Build history of the part. All positions in model axes, mm. A direction names the side the tool comes from. Round coordinates to 2 decimals unless told otherwise and drop trailing zeros. Order: outer loops, then holes, each group sorted by start corner. A loop starts at its lowest first (then second) coordinate and runs counter-clockwise, first axis right, second up. Notation, with made-up numbers: M 9.5,8.25 L 63.5,8.25 A32 cw 63.5,44.25 Z; hole C 8,-21 d2. An arc over 180 degrees is marked long. One line per item, written item: value. Start each with the question number.
Item 1: Band-saw the part on C-C, the plane z = 10.5. Give the number of separate pieces and of enclosed holes in the cut face, then the cut area to 3 significant figures.
Item 2: Tool access for faces 4 (the flat face through (19, -16, 9.525)), 5 (the flat face through (27.99, -7.01, 35.22)), 6 (the flat face through (12.7, -8, 23)): list every direction of +Z, -Z, +X, -X, +Y, -Y with a clear straight run to the whole face (end or side of a thin tool).
Item 3: Band-saw the part on B-B, the plane z = 5.5. Write the cut outline in (x, y).
Item 4: Two-plate mould, pull along X, no slides. Class faces 1 (the flat face through (11.1, -22.23, 26.97)), 2 (the flat face through (12.7, -15, 21)), 3 (the flat face through (14, -32.4, 15.8)): +X half, -X half, draft (parallel to the pull), parting line (faces both ways), or undercut.
Item 5: Probe L1, parallel to X at y = -7.5, z = 15; L2, parallel to Y at x = 10.5, z = 24.5; L3, parallel to Y at x = 13, z = 28. List the from-to ranges inside material, lowest first.
Item 6: Band-saw the part on A-A, the plane x = 3.5. Write the cut outline in (y, z) (3 decimals).
Item 7: Band-saw the part on D-D, the plane y = -32.5. Write the cut outline in (x, z) (3 decimals).
Item 8: Pin check, flat tips, straight feed: pin 1 (3 mm diameter, centred on x = 20.5, y = -32.5, fed in from -Z) (3 decimals); pin 2 (1 mm diameter, centred on y = -31.5, z = 13, fed in from -X); pin 3 (2.5 mm diameter, centred on y = -28.5, z = 27.5, fed in from -X); pin 4 (10 mm diameter, centred on x = 28.5, y = -24, fed in from -Z). Stop position of each tip, or through.
```python
from build123d import *

# Parameters (mm, degrees)
F0_W      = 38.1
F0_H      = 37.973095
F1_DEPTH  = 38.1
F6_DEPTH  = 38.1
F8_DEPTH  = 38.1
F9_W      = 25.4
F9_H      = 7.62
F10_DEPTH = 38.1


with BuildPart() as f1:
    # F0 (on Front) → F1 (new body)
    with BuildSketch(Plane.XZ):
        with Locations((19.05, 18.986548)):
            Rectangle(F0_W, F0_H)
    extrude(amount=F1_DEPTH)

    # F5 (on offset) → F6 (cut)
    with BuildSketch(Plane.YZ.offset(38.1)):
        Polygon((-11.43, 15.875), (-6.35, 38.1), (-31.75, 38.1), (-26.67, 15.875), (-21.59, 28.575), (-16.51, 28.575), align=None)
        Polygon((-6.35, 0), (0, 0), (0, 38.1), align=None)
        Polygon((-25.4, 0), (-12.7, 0), (-19.05, 15.875), align=None)
        Polygon((-31.75, 0), (-38.1, 38.1), (-38.1, 0), align=None)
    extrude(amount=-F6_DEPTH, mode=Mode.SUBTRACT)

    # F7 (on offset) → F8 (cut)
    with BuildSketch(Plane.XZ.offset(38.1)):
        Polygon((11.43, 22.225), (6.35, 0), (31.75, 0), (26.67, 22.225), (21.59, 9.525), (16.51, 9.525), align=None)
        Polygon((25.4, 38.1), (12.7, 38.1), (19.05, 22.225), align=None)
        Polygon((31.75, 38.1), (38.1, 0), (38.1, 38.1), align=None)
        Polygon((0, 38.1), (0, 0), (6.35, 38.1), align=None)
    extrude(amount=-F8_DEPTH, mode=Mode.SUBTRACT)

    # F9 (on offset) → F10 (cut)
    with BuildSketch(Plane.XY.offset(38.1)):
        with Locations((25.4, -11.43)):
            Rectangle(F9_W, F9_H)
        with Locations((12.7, -26.67)):
            Rectangle(F9_W, F9_H)
    extrude(amount=-F10_DEPTH, mode=Mode.SUBTRACT)


solid = f1.part
```
Output:
1. separate pieces: 10
1. enclosed holes: 0
1. area: 293 mm²
2. face 4: -Z, +Y, -Y
2. face 5: +Z, +X, -X
2. face 6: +Z, -Z, +X
3. outline: M 0.92,-32.67 L 7.61,-32.67 L 7.61,-30.48 L 0.92,-30.48 Z; M 0.92,-14.9 L 7.61,-14.9 L 7.61,-5.43 L 0.92,-5.43 Z; M 30.49,-32.67 L 37.18,-32.67 L 37.18,-23.2 L 30.49,-23.2 Z; M 30.49,-7.62 L 37.18,-7.62 L 37.18,-5.43 L 30.49,-5.43 Z
4. face 1: draft
4. face 2: +X half
4. face 3: undercut
5. L1: x = 2.5 to 9.78, 14.32 to 23.78, 28.32 to 35.6
5. L2: y = -35.83 to -30.48, -22.86 to -14.88, -9.46 to -2.27
5. L3: y = -36.42 to -30.48, -21.82 to -16.28, -7.62 to -1.68
6. outline: M -35.25,21 L -31.75,0 L -30.48,0 L -30.48,21 Z; M -22.86,6.35 L -19.05,15.875 L -12.7,0 L -6.35,0 L -2.85,21 L -10.259,21 L -11.43,15.875 L -13.48,21 L -22.86,21 Z
7. outline: M 0.75,4.5 L 7.379,4.5 L 11.43,22.225 L 16.51,9.525 L 21.59,9.525 L 26.67,22.225 L 30.721,4.5 L 37.35,4.5 L 31.771,37.973 L 25.349,37.973 L 19.05,22.225 L 12.751,37.973 L 6.329,37.973 Z
8. pin 1: stops at z = 9.525
8. pin 2: stops at x = 2.08
8. pin 3: stops at x = 25.4
8. pin 4: stops at z = 0
